Work out the finished part from the listing and answer in its coordinate system (mm). A direction names the side the tool comes from. Coordinates: 2 decimals unless noted, no trailing zeros. Order: outer loops, then holes, each group sorted by start corner. A loop starts at its lowest first (then second) coordinate and runs counter-clockwise, first axis right, second up.
1. The part is cut by section A-A, the plane x = -7. Give the vertices of the cut face in (y, z).
2. Flat-ended cylindrical pins translate along their axes: pin 1 Ø6.5 at (x, y) = (7, 6.76) entering from +Z; pin 2 Ø1.6 at (x, z) = (0.5, 4.5) entering from +Y; pin 3 Ø1 at (x, z) = (4, 3) entering from -Y; pin 4 Ø3 at (x, y) = (1, 7) entering from -Z. Find the tip coordinate at first contact, or state that the pin passes through.
3. The part is cut by section C-C, the plane x = 12.5. Give the vertices of the cut face in (y, z).
4. The part is cut by section D-D, the plane y = 2. Give the vertices of the cut face in (x, z).
5. A tool of negligible diameter and unlimited length cuts with its end or side. For faces 4 (the flat face through (-7.6, 4.45, 3.99)), 5 (the cylindrical face through (8.18, 5.68, 3.79)), 6 (the flat face through (0, 11.66, 4)), 7 (the flat face through (0, 11, 0)), 8 (the cylindrical face through (11.026, 7.809, 1.479)), from which of +Z, -Z, +X, -X, +Y, -Y can it reach the whole face along a straight path? Write none if from no direction.
6. Find the intervals of material crossed by probe 1 along X at (y, z) = (9.25, 0.3); probe 2 along X at (y, z) = (6.75, 1.4); probe 3 along X at (y, z) = (6.5, 4.3), in increasing order.
7. Determine the mould class of faces 1 (the flat face through (-15, 9, 2)), 2 (the flat face through (0.21, 12.057, 1.521)), 3 (the cylindrical face through (-13.974, 7.809, 1.479)) for opening direction X: +X half, -X half, draft (parallel to the pull), parting line (faces both ways), or undercut.
8. The part is cut by section B-B, the plane z = 1.7. Give the vertices of the cut face in (x, y), then the cut area to 3 significant figures.
```python
from build123d import *

# Parameters (mm, degrees)
RESSALTO_EXTRUS_O1_DEPTH   = 3
CHANFRO1_SIZE              = 5
CHANFRO1_SIZE_2            = 2.331538291
CHANFRO2_SIZE              = 1.339745962
CHANFRO2_SIZE_2            = 5
RESSALTO_EXTRUS_O2_DEPTH   = 2
CORTE_EXTRUS_O1_DEPTH      = 21.133400832
CORTE_EXTRUS_O1_DEPTH_BACK = 21.133400832
ESBO_O3_R                  = 1.6
ESBO_O4_R                  = 2
CORTE_EXTRUS_O2_DEPTH      = 3
ESBO_O6_W                  = 5.6
ESBO_O6_H                  = 6
CORTE_EXTRUS_O3_DEPTH      = 2
CHANFRO3_SIZE              = 0.4


with BuildPart() as part:
    # Esboço1 → Ressalto-extrusão1 (new body)
    with BuildSketch(Plane.XY):
        Polygon((-15, 13), (-15, 4.019237886), (0, 0), (15, 4.019237886), (15, 13), align=None)
    extrude(amount=RESSALTO_EXTRUS_O1_DEPTH)

    # Chanfro1
    # the kernel refuses this chamfer: 5, 2.331538291 mm, written as the material it takes off along each edge
    with BuildSketch(Plane(origin=(-27.513450616, 7.372206873, 3), x_dir=(-0.00422163992492442, -0.015755374691079384, -0.9998669641130704), z_dir=(0.9659258262890691, -0.25881904510251785, 0)), Plane(origin=(-12.513450616, -3.352968987, 3), x_dir=(0.004221639924924417, -0.015755374691079373, -0.9998669641130704), z_dir=(0.9659258262890691, 0.25881904510251785, 0))) as chanfro1_piece_1:
        Polygon((CHANFRO1_SIZE * 0.999866964113, CHANFRO1_SIZE * 0.0163111641311), (-CHANFRO1_SIZE_2 * 0.0163111641295, CHANFRO1_SIZE_2 * 0.999866964017), (0, 0), align=None)
    extrude(amount=41.43889742, mode=Mode.SUBTRACT)

    # Chanfro2
    # the kernel refuses this chamfer: 5, 1.339745962 mm, written as the material it takes off along each edge
    with BuildSketch(Plane(origin=(27.983607851, 13, 3), x_dir=(0, -0.9905000388259543, 0.13751244702128929), z_dir=(-1, 0, 0))) as chanfro2_piece_1:
        Polygon((CHANFRO2_SIZE * 0.990500038941, -CHANFRO2_SIZE * 0.137512447037), (-CHANFRO2_SIZE_2 * 0.137512447021, -CHANFRO2_SIZE_2 * 0.990500038826), (0, 0), align=None)
    extrude(amount=55.967215702, mode=Mode.SUBTRACT)

    # Esboço2 → Ressalto-extrusão2 (add)
    with BuildSketch(Plane.XY.offset(3)):
        Polygon((0, 2.413786056), (15, 6.433023943), (15, 11.660254038), (-15, 11.660254038), (-15, 6.433023943), align=None)
    extrude(amount=RESSALTO_EXTRUS_O2_DEPTH)

    # Esboço3 → Corte-extrusão1 (cut, two sides: drawn at the far end of the back side and taken through both)
    with BuildSketch(Plane.XY.offset(-CORTE_EXTRUS_O1_DEPTH_BACK)):
        with Locations((-7, 6.762338276)):
            Circle(ESBO_O3_R)
        with Locations(Location((7, 6.762338276, 0), (0, 0, 180))):
            Circle(ESBO_O3_R)
        with Locations((-12.5, 9.160254038)):
            Circle(ESBO_O3_R)
        with Locations(Location((12.5, 9.160254038, 0), (0, 0, 180))):
            Circle(ESBO_O3_R)
    extrude(amount=CORTE_EXTRUS_O1_DEPTH + CORTE_EXTRUS_O1_DEPTH_BACK, mode=Mode.SUBTRACT)

    # Esboço4 → Corte-extrusão2 (cut)
    with BuildSketch(Plane(origin=(0, 0, 0), x_dir=(-1, 0, 0), z_dir=(0, 0, -1))):
        with Locations(Location((-7, 6.762338276, 0), (0, 0, 180))):
            Circle(ESBO_O4_R)
        with Locations(Location((12.5, 9.160254038, 0), (0, 0, 180))):
            Circle(ESBO_O4_R)
        with Locations(Location((-12.5, 9.160254038, 0), (0, 0, 180))):
            Circle(ESBO_O4_R)
        with Locations(Location((7, 6.762338276, 0), (0, 0, 180))):
            Circle(ESBO_O4_R)
    extrude(amount=-CORTE_EXTRUS_O2_DEPTH, mode=Mode.SUBTRACT)

    # Esboço6 → Corte-extrusão3 (cut)
    with BuildSketch(Plane(origin=(0, 0, 0), x_dir=(-1, 0, 0), z_dir=(0, 0, -1))):
        with Locations((0, 7)):
            Rectangle(ESBO_O6_W, ESBO_O6_H)
    extrude(amount=-CORTE_EXTRUS_O3_DEPTH, mode=Mode.SUBTRACT)

    # Chanfro3
    chanfro3_edges = [part.edges().sort_by_distance(p)[0] for p in [
        (14.1, 9.160254038, 5),
        (-14.1, 9.160254038, 5),
        (8.6, 6.762338276, 5),
        (-8.6, 6.762338276, 5),
    ]]
    chamfer(chanfro3_edges, length=CHANFRO3_SIZE)


solid = part.part
```
Geometry says:
1. outline: (2.84, 0) - (4.76, 0) - (4.76, 3) - (5.16, 3) - (5.16, 4.6) - (4.76, 5) - (4.29, 5) - (4.29, 3) - close; (8.36, 3) - (8.76, 3) - (8.76, 0) - (12.46, 0) - (11.66, 3) - (11.66, 5) - (8.76, 5) - (8.36, 4.6) - close
2. pin 1: stops at z = 5
2. pin 2: stops at y = 11.66
2. pin 3: stops at y = 3.21
2. pin 4: stops at z = 2
3. outline: (4.31, 0) - (7.16, 0) - (7.16, 3) - (7.56, 3) - (7.56, 4.6) - (7.16, 5) - (5.76, 5) - (5.76, 3) - close; (10.76, 3) - (11.16, 3) - (11.16, 0) - (12.46, 0) - (11.66, 3) - (11.66, 5) - (11.16, 5) - (10.76, 4.6) - close
4. outline: (-3.86, 0) - (3.86, 0) - (0, 2.14) - close
5. face 4: +Z, -X, -Y
5. face 5: +Z, -Z
5. face 6: +Z, +X, -X, +Y
5. face 7: -Z, +X, -X, +Y, -Y
5. face 8: -Z
6. probe 1: x = -15 to -14.5, -10.5 to -2.8, 2.8 to 10.5, 14.5 to 15
6. probe 2: x = -15 to -9, -5 to -2.8, 2.8 to 5, 9 to 15
6. probe 3: x = -15 to -8.58, -5.42 to 5.42, 8.58 to 15
7. face 1: -X half
7. face 2: draft
7. face 3: undercut
8. outline: (-15, 5.81) - (0, 1.79) - (15, 5.81) - (15, 12.01) - (-15, 12.01) - close; hole circle Ø4 at (-12.5, 9.16); hole circle Ø4 at (-7, 6.76); hole (-2.8, 4) - (2.8, 4) - (2.8, 10) - (-2.8, 10) - close; hole circle Ø4 at (7, 6.76); hole circle Ø4 at (12.5, 9.16)
8. area: 163 mm2
